Could you check a few things on this model? Use its own coordinates, in mm. A direction names the side the tool comes from. Round coordinates to 2 decimals unless told otherwise and drop trailing zeros. Loops run counter-clockwise (first coordinate to the right, second up) from the corner with the lowest first, then second, coordinate; pieces in that order, holes last. Notation, with made-up numbers: (35, -17) - (76, -17) arc R13 ccw to (76, -9) - close; hole circle Ø4 at (79, 23.5). An arc over 180 degrees is marked (long way). Answer as CSV lines item,"result". Start each with the question number.
1) Which directions (+Z, -Z, +X, -X, +Y, -Y) give clear straight access to the entire face, cutting with the end or side of a thin tool? Please do faces 1 (the face through (9.55, 0.27, 9.57)), 2 (the face through (4.39, -0.27, 5.45)), 3 (the face through (-9, 0, -2.63)), 4 (the face through (9, 0, 2.63)).
2) We'd pull the mould along X, two halves only. Please class faces 5 (the face through (10, 0, 6)), 6 (the face through (5.41, -0.27, 4.35)), 7 (the face through (-0.1, -19.05, -2.4)): pulls with the +X half, pulls with the -X half, needs draft (parallel to the pull), parting line crosses it, or undercut.
3) Please list where these lines run through material, in increasing order: line 1 along X through (y, z) = (-13.75, 0); line 2 along X through (y, z) = (-14, 4.75); line 3 along Z through (x, y) = (-4.5, 16.5).
4) Suppose I cut it at B-B, the plane z = 0. Write out the boundary of the cut face in (x, y).
5) Suppose I cut it at A-A, the plane z = 7.5. Write out the boundary of the cut face in (x, y).
6) Suppose I cut it at D-D, the plane z = 4.5. Write out the boundary of the cut face in (x, y), then the cut area to 3 significant figures.
7) I'm going to push a flat-ended pin straight in: pin 1 Ø1.6 at (y, z) = (-6, 9.5) entering from -X. Where does the tip first touch, or does it pass through?
8) Suppose I cut it at C-C, the plane x = 0. Write out the boundary of the cut face in (y, z), then the cut area to 3 significant figures.
```python
from build123d import *

# Parameters (mm, degrees)
BOSS_EXTRUDE1_DEPTH     = 19.05
CUT_EXTRUDE5_DEPTH      = 24.725566379
CUT_EXTRUDE5_DEPTH_BACK = 24.725566379
SKETCH5_R               = 2.1
CUT_EXTRUDE6_DEPTH      = 13
CUT_EXTRUDE7_START      = -13
SKETCH4_R               = 2.1
CUT_EXTRUDE7_DEPTH      = 13


with BuildPart() as part:
    # Sketch1 → Boss-Extrude1 (new, symmetric)
    with BuildSketch(Plane(origin=(0, 0, 0), x_dir=(1, 0, 0), z_dir=(0, 1, 0))):
        with BuildLine():
            Line((-8.5, -10), (8.5, -10))
            ThreePointArc((8.5, -10), (9.560660172, -9.560660172), (10, -8.5))
            Line((10, -8.5), (10, 8.5))
            ThreePointArc((10, 8.5), (9.560660172, 9.560660172), (8.5, 10))
            Line((8.5, 10), (-8.5, 10))
            ThreePointArc((-8.5, 10), (-9.560660172, 9.560660172), (-10, 8.5))
            Line((-10, 8.5), (-10, -8.5))
            ThreePointArc((-10, -8.5), (-9.560660172, -9.560660172), (-8.5, -10))
        make_face()
    extrude(amount=BOSS_EXTRUDE1_DEPTH, both=True)

    # Sketch3 → Cut-Extrude5 (cut, two sides: drawn at the far end of the back side and taken through both)
    with BuildSketch(Plane(origin=(0, 0, 0), x_dir=(1, 0, 0), z_dir=(0, 1, 0)).offset(-CUT_EXTRUDE5_DEPTH_BACK)):
        Polygon((2.63, 10), (-2.63, 10), (-2.63, 8.5), (-6, 8.5), (-6, 7.060660172), (-2.739339828, 3.8), (2.739339828, 3.8), (6, 7.060660172), (6, 8.5), (2.63, 8.5), align=None)
        Polygon((10, -2.63), (10, 2.63), (8.5, 2.63), (8.5, 6), (7.060660172, 6), (3.8, 2.739339828), (3.8, -2.739339828), (7.060660172, -6), (8.5, -6), (8.5, -2.63), align=None)
        Polygon((-2.63, -10), (2.63, -10), (2.63, -8.5), (6, -8.5), (6, -7.060660172), (2.739339828, -3.8), (-2.739339828, -3.8), (-6, -7.060660172), (-6, -8.5), (-2.63, -8.5), align=None)
        Polygon((-10, 2.63), (-10, -2.63), (-8.5, -2.63), (-8.5, -6), (-7.060660172, -6), (-3.8, -2.739339828), (-3.8, 2.739339828), (-7.060660172, 6), (-8.5, 6), (-8.5, 2.63), align=None)
    extrude(amount=CUT_EXTRUDE5_DEPTH + CUT_EXTRUDE5_DEPTH_BACK, mode=Mode.SUBTRACT)

    # Sketch5 → Cut-Extrude6 (cut)
    with BuildSketch(Plane.XZ.offset(19.05)):
        with Locations(Location((0, 0, 0), (0, 0, 270))):
            Circle(SKETCH5_R)
    extrude(amount=-CUT_EXTRUDE6_DEPTH, mode=Mode.SUBTRACT)

    # Sketch4 → Cut-Extrude7 (cut)
    with BuildSketch(Plane(origin=(0, 19.05, 0), x_dir=(1, 0, 0), z_dir=(0, 1, 0)).offset(CUT_EXTRUDE7_START)):
        with Locations(Location((0, 0, 0), (0, 0, 90))):
            Circle(SKETCH4_R)
    extrude(amount=CUT_EXTRUDE7_DEPTH, mode=Mode.SUBTRACT)


solid = part.part
```
Filled sheet:
1,face 1,"+Z, +X, +Y, -Y"
1,face 2,"+Y, -Y"
1,face 3,"-X, +Y, -Y"
1,face 4,"+X, +Y, -Y"
2,face 5,"pulls with the +X half"
2,face 6,"undercut"
2,face 7,"needs draft"
3,line 1,"-3.8 to -2.1, 2.1 to 3.8"
3,line 2,"-10 to -8.5, -5.81 to -3.69, 3.69 to 5.81, 8.5 to 10"
3,line 3,"-10 to -8.5, -5.56 to -3.44, 3.44 to 5.56, 8.5 to 10"
4,outline,"(-3.8, -19.05) - (-2.1, -19.05) - (-2.1, -6.05) - (2.1, -6.05) - (2.1, -19.05) - (3.8, -19.05) - (3.8, 19.05) - (2.1, 19.05) - (2.1, 6.05) - (-2.1, 6.05) - (-2.1, 19.05) - (-3.8, 19.05) - close"
5,outline,"(-10, -19.05) - (-6, -19.05) - (-6, 19.05) - (-10, 19.05) - close; (6, -19.05) - (10, -19.05) - (10, 19.05) - (6, 19.05) - close"
6,outline,"(-10, -19.05) - (-8.5, -19.05) - (-8.5, 19.05) - (-10, 19.05) - close; (-5.56, -19.05) - (-3.44, -19.05) - (-3.44, 19.05) - (-5.56, 19.05) - close; (3.44, -19.05) - (5.56, -19.05) - (5.56, 19.05) - (3.44, 19.05) - close; (8.5, -19.05) - (10, -19.05) - (10, 19.05) - (8.5, 19.05) - close"
6,area,"276 mm²"
7,pin 1,"x = -9.99"
8,outline,"(-19.05, -3.8) - (19.05, -3.8) - (19.05, -2.1) - (6.05, -2.1) - (6.05, 2.1) - (19.05, 2.1) - (19.05, 3.8) - (-19.05, 3.8) - (-19.05, 2.1) - (-6.05, 2.1) - (-6.05, -2.1) - (-19.05, -2.1) - close"
8,area,"180 mm²"
